Can you work these out from the model? Positions are in its coordinate system, mm. A direction names the side the tool comes from. Give positions to 0.01 mm unless a question says otherwise; leave off trailing zeros. Write each loop counter-clockwise with the first axis right and the second up, starting at its lowest first coordinate (ties: lowest second). Pieces come first, ordered by that corner, then holes. Notation, with made-up numbers: (12.5, 27.25) -> (18.5, 27.25) arc R13 ccw to (18.5, 37.25) -> close; hole circle Ø8 at (88.5, 61.25). An arc over 180 degrees is marked (long way). Answer as CSV lines item,"result". Start each with the question number.
1. I need wall thicknesses on line 1 (Y direction, x = 0, z = 4); line 2 (Y direction, x = 0, z = 8.9); line 3 (X direction, y = -20, z = 4). Which ranges of each line are inside material? Lowest first, please. Write a range as [from, to].
2. If we section it at D-D on x = 8.5: Write out the boundary of the cut face in (y, z), plus the area to 3 significant figures.
3. If we section it at B-B on x = 0: Write out the boundary of the cut face in (y, z), plus the area to 3 significant figures.
4. If we section it at C-C on z = 8.75: Write out the boundary of the cut face in (x, y).
5. If we mould it in two halves opening along X, with no side actions, what happens to faces 1 (the face through (-1.302, -10.085, 10.235)), 2 (the face through (25.4, -1, 6)), 3 (the face through (0, 1, 0))? For each: pulls with the +X half, pulls with the -X half, needs draft (parallel to the pull), parting line crosses it, or undercut.
6. If we section it at A-A on y = -20: Write out the boundary of the cut face in (x, z), plus the area to 3 significant figures.
7. I'm going to push flat-ended pins straight in: P1, Ø10.5, axis at x = 0, y = -20, coming from the -Z side; P2, Ø12, axis at x = 0, y = -20, coming from the +Z side. Where does each tip first touch, or does it pass through?
8. On a 3-axis mill with a long thin cutter (end or side, diameter ignored), from which of +Z, -Z, +X, -X, +Y, -Y can I reach the whole of each face in a straight line? I mean faces 4 (the face through (0, 1, 12.7)), 5 (the face through (-0.1, -24.3, 7.7)). Say none if no direction works.
```python
from build123d import *

# Parameters (mm, degrees)
CROQUIS1_W              = 50.8
CROQUIS1_H              = 80
CROQUIS1_R              = 4
SALIENTE_EXTRUIR1_DEPTH = 12.7
CROQUIS2_R              = 10
CORTAR_EXTRUIR1_DEPTH   = 5


with BuildPart() as part:
    # Croquis1 → Saliente-Extruir1 (new body)
    with BuildSketch(Plane.XY):
        Rectangle(CROQUIS1_W, CROQUIS1_H)
        with Locations((0, -20)):
            Circle(CROQUIS1_R, mode=Mode.SUBTRACT)
    extrude(amount=SALIENTE_EXTRUIR1_DEPTH)

    # Croquis2 → Cortar-Extruir1 (cut)
    with BuildSketch(Plane.XY.offset(12.7)):
        with Locations((0, -20)):
            Circle(CROQUIS2_R)
    extrude(amount=-CORTAR_EXTRUIR1_DEPTH, mode=Mode.SUBTRACT)


solid = part.part
```
Computed values:
1,line 1,"y = [-40, -24], [-16, 40]"
1,line 2,"y = [-40, -30], [-10, 40]"
1,line 3,"x = [-25.4, -4], [4, 25.4]"
2,outline,"(-40, 0) -> (40, 0) -> (40, 12.7) -> (-14.73, 12.7) -> (-14.73, 7.7) -> (-25.27, 7.7) -> (-25.27, 12.7) -> (-40, 12.7) -> close"
2,area,"963 mm2"
3,outline,"(-40, 0) -> (-24, 0) -> (-24, 7.7) -> (-30, 7.7) -> (-30, 12.7) -> (-40, 12.7) -> close; (-16, 0) -> (40, 0) -> (40, 12.7) -> (-10, 12.7) -> (-10, 7.7) -> (-16, 7.7) -> close"
3,area,"854 mm2"
4,outline,"(-25.4, -40) -> (25.4, -40) -> (25.4, 40) -> (-25.4, 40) -> close; hole circle Ø20 at (0, -20)"
5,face 1,"undercut"
5,face 2,"pulls with the +X half"
5,face 3,"needs draft"
6,outline,"(-25.4, 0) -> (-4, 0) -> (-4, 7.7) -> (-10, 7.7) -> (-10, 12.7) -> (-25.4, 12.7) -> close; (4, 0) -> (25.4, 0) -> (25.4, 12.7) -> (10, 12.7) -> (10, 7.7) -> (4, 7.7) -> close"
6,area,"484 mm2"
7,P1,"stops at z = 0"
7,P2,"stops at z = 7.7"
8,face 4,"+Z, +X, -X, +Y, -Y"
8,face 5,"+Z"
